from build123d import *

# Parameters (mm, degrees)
F0_R      = 1.5
F1_DEPTH  = 10
F0_R_2    = 2.85
F1_FACE_R = 1.5
F2_DEPTH  = 1.65
F4_DEPTH  = 1
F5_R      = 1.5


with BuildPart() as f1:
    # F0 (on Top) → F1 (new body)
    with BuildSketch(Plane.XY):
        Circle(F0_R)
    extrude(amount=-F1_DEPTH)

    # F0 (on Top) + F1_face (on face) → F2 (join)
    with BuildSketch(Plane.XY):
        Circle(F0_R_2)
        Circle(F0_R, mode=Mode.SUBTRACT)
    with BuildSketch(Plane.XY):
        Circle(F1_FACE_R)
    extrude(amount=F2_DEPTH)

    # F3 (on face) → F4 (cut)
    with BuildSketch(Plane.XY.offset(1.65)):
        Polygon((0, 1.1547005384), (-1, 0.5773502692), (-1, -0.5773502692), (0, -1.1547005384), (1, -0.5773502692), (1, 0.5773502692), align=None)
    extrude(amount=-F4_DEPTH, mode=Mode.SUBTRACT)

    # F5
    f5_edges = [f1.edges().sort_by_distance(p)[0] for p in [
        (-2.85, 0, 1.65),
    ]]
    fillet(f5_edges, radius=F5_R)


solid = f1.part
For this review, take the finished solid that the model builds, in its own axes (mm). A direction names the side the tool comes from. Round coordinates to 2 decimals unless told otherwise and drop trailing zeros. Loops run counter-clockwise (first coordinate to the right, second up) from the corner with the lowest first, then second, coordinate; pieces in that order, holes last. Notation, with made-up numbers: (-16, 12) - (4, 12) arc R30 cw to (4, 44) - close; hole circle Ø7 at (17.5, 9). An arc over 180 degrees is marked (long way). Use one line per item in the form item = value.
1) Tool access review of faces 5 (the face through (-1, 0, 1)), 6 (the face through (0, 0, -10)): name each direction out of +Z, -Z, +X, -X, +Y, -Y from which nothing blocks a thin tool from reaching the whole face with its end or side.
Solutions:
face_5 = +Z
face_6 = -Z, +X, -X, +Y, -Y
2) Mouldability with a two-part tool opening along Y and no side actions: class faces 1 (the face through (0, 0, 0.65)), 2 (the face through (-1.5, 0.07, -4.93)), 3 (the face through (0.49, -0.87, 1.16)), 4 (the face through (1.2, -1.2, 0)) as pulls with the +Y half, pulls with the -Y half, needs draft (parallel to the pull), parting line crosses it, or undercut.
Solutions:
face_1 = undercut
face_2 = parting line crosses it
face_3 = undercut
face_4 = needs draft
3) Wall thickness on probe 1 along Z at (x, y) = (1.35, -0.45); probe 2 along Z at (x, y) = (-0.1, 0.35); probe 3 along X at (y, z) = (0.9, -5.25): over which ranges is each line inside the solid? List them lowest first.
Solutions:
probe_1 = -10 to 1.65
probe_2 = -10 to 0.65
probe_3 = -1.2 to 1.2
4) Clearance check with flat-ended pins moving along their axes: P1, Ø0.5, axis at y = 0, z = 1, coming from the +X side; P2, Ø2, axis at y = 0, z = -8.5, coming from the +X side; P3, Ø1.1, axis at y = 0, z = 1.5, coming from the -X side. State where each tip first meets the part, or that it passes through.
Solutions:
P1 = 2.72
P2 = 1.5
P3 = -2.62
5) We need section A-A on z = -3.5. Write out the cut boundary in (x, y), then the cut area to 3 significant figures.
Solutions:
outline = circle Ø3 at (0, 0)
area = 7.07 mm2
